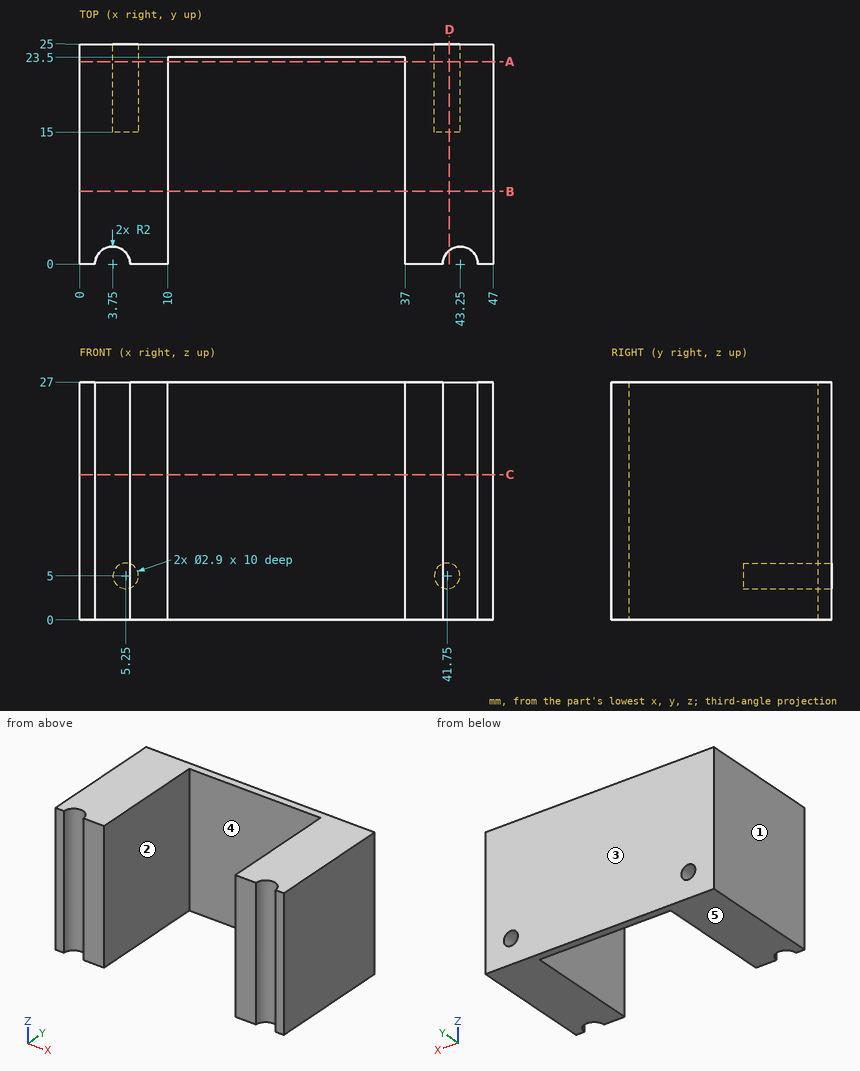
Check sheet for the drawn part. Datum: minimum x, y, z corner. Units: mm. A direction names the side the tool comes from. Round coordinates to 2 decimals unless told otherwise and drop trailing zeros. Loops run counter-clockwise (first coordinate to the right, second up) from the corner with the lowest first, then second, coordinate; pieces in that order, holes last.
Item 1: Cross-section at D-D on x = 42. Record the boundary of the cut face in (y, z).
Item 2: Cross-section at C-C on z = 16.5. Record the boundary of the cut face in (x, y), then the cut area to 3 significant figures.
Item 3: Cross-section at B-B on y = 8.25. Record the boundary of the cut face in (x, z).
Item 4: Access from +Z, -Z, +X, -X, +Y, -Y to the whole of each face (thin tool, end or side, straight path). Record for the marked faces 4 and 5.
Item 5: Gauge pin test, flat ends, axial feed: pin 1 (1.5 mm diameter, centred on x = 37, y = 4, fed in from -Z); pin 2 (1.5 mm diameter, centred on x = 5, z = 4.5, fed in from +Y). Record the tip position at first contact, or that the pin passes through.
Item 6: Mould release check, pull along X, two halves, no side actions. Record for the marked faces 1, 2 and 3: pulls with the +X half, pulls with the -X half, needs draft (parallel to the pull), parting line crosses it, or undercut.
Item 7: Thickness scan on line 1 (X direction, y = 20.75, z = 19.5); line 2 (Z direction, x = 41.75, y = 20.5); line 3 (Y direction, x = 36, z = 12). Record the ranges inside material, lowest first.
Item 8: Cross-section at A-A on y = 23. Record the boundary of the cut face in (x, z), then the cut area to 3 significant figures.
Answer sheet:
1. outline: (1.56, 0) - (25, 0) - (25, 3.57) - (15, 3.57) - (15, 6.43) - (25, 6.43) - (25, 27) - (1.56, 27) - close
2. outline: (0, 0) - (1.75, 0) arc R2 cw to (5.75, 0) - (10, 0) - (10, 23.5) - (37, 23.5) - (37, 0) - (41.25, 0) arc R2 cw to (45.25, 0) - (47, 0) - (47, 25) - (0, 25) - close
2. area: 528 mm2
3. outline: (0, 0) - (10, 0) - (10, 27) - (0, 27) - close; (37, 0) - (47, 0) - (47, 27) - (37, 27) - close
4. face 4: +Z, -Z, -Y
4. face 5: -Z, +X, -X, +Y, -Y
5. pin 1: stops at z = 0
5. pin 2: stops at y = 15
6. face 1: pulls with the -X half
6. face 2: undercut
6. face 3: needs draft
7. line 1: x = 0 to 10, 37 to 47
7. line 2: z = 0 to 3.55, 6.45 to 27
7. line 3: y = 23.5 to 25
8. outline: (0, 0) - (10, 0) - (10, 27) - (0, 27) - close; (37, 0) - (47, 0) - (47, 27) - (37, 27) - close; hole circle Ø2.9 at (5.25, 5); hole circle Ø2.9 at (41.75, 5)
8. area: 527 mm2
